Check sheet for the drawn part. Datum: minimum x, y, z corner. Units: mm. Coordinates: 2 decimals unless noted, no trailing zeros. Order: outer loops, then holes, each group sorted by start corner. A loop starts at its lowest first (then second) coordinate and runs counter-clockwise, first axis right, second up. Notation, with made-up numbers: M 30.5,65.5 L 47.5,65.5 A23 ccw 47.5,95.5 Z; hole C -15.5,46.5 d3. An arc over 180 degrees is marked long. Return JSON: item names as keys, results as strings. Group by question number.
Q1. Section check A-A, the plane x = 30. Enter the section's corners in (y, z).
Q2. Section check C-C, the plane x = 6. Enter the section's corners in (y, z), then the cut area to 3 significant figures.
Q3. Section check B-B, the plane y = 30. Enter the section's corners in (x, z), then the cut area to 3 significant figures.
Q4. Go/stop test with flat-tipped pins: pin 1 Ø1 at (y, z) = (42, 1.5) entering from -X; pin 2 Ø0.6 at (y, z) = (40, 1.5) entering from -X; pin 3 Ø1 at (x, z) = (24.5, 1) entering from -Y; pin 4 Ø3 at (x, y) = (6, 30) entering from -Z. Record where each tip stops, or that it passes through.
Q5. Thickness scan on probe 1 along Y at (x, z) = (41, 1); probe 2 along X at (y, z) = (39, 1); probe 3 along Y at (x, z) = (39, 0.3). Record the ranges inside material, lowest first.
Q6. Section check D-D, the plane z = 0.4. Enter the section's corners in (x, y).
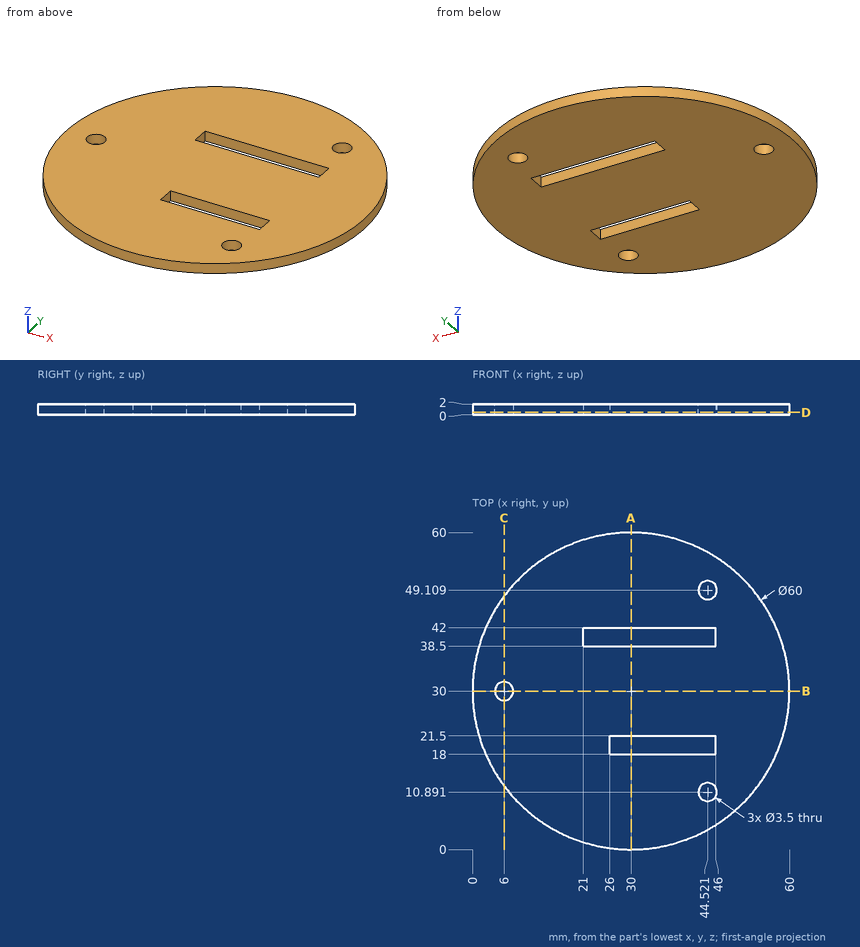
Numbers:
{
 "1": {"outline": "M 0,0 L 18,0 L 18,2 L 0,2 Z; M 21.5,0 L 38.5,0 L 38.5,2 L 21.5,2 Z; M 42,0 L 60,0 L 60,2 L 42,2 Z"},
 "2": {"outline": "M 12,0 L 28.25,0 L 28.25,2 L 12,2 Z; M 31.75,0 L 48,0 L 48,2 L 31.75,2 Z", "area": "65.0 mm2"},
 "3": {"outline": "M 0,0 L 4.25,0 L 4.25,2 L 0,2 Z; M 7.75,0 L 60,0 L 60,2 L 7.75,2 Z", "area": "113 mm2"},
 "4": {"pin 1": "stops at x = 2.29", "pin 2": "stops at x = 1.61", "pin 3": "stops at y = 0.42", "pin 4": "passes through"},
 "5": {"probe 1": "y = 2.09 to 18, 21.5 to 38.5, 42 to 57.91", "probe 2": "x = 1.38 to 21, 46 to 58.62", "probe 3": "y = 1.38 to 18, 21.5 to 38.5, 42 to 58.62"},
 "6": {"outline": "C 30,30 d60; hole C 6,30 d3.5; hole M 21,38.5 L 46,38.5 L 46,42 L 21,42 Z; hole M 26,18 L 46,18 L 46,21.5 L 26,21.5 Z; hole C 44.52,10.89 d3.5; hole C 44.52,49.11 d3.5"}
}
